CAD build for the part. Positions are in the model's coordinates, mm. Face numbers are marked on the shaded views. A direction names the side the tool comes from. Give positions to 0.01 mm unless a question says otherwise; leave off trailing zeros. Write each loop counter-clockwise with the first axis right and the second up, starting at its lowest first coordinate (ties: lowest second). Pieces come first, ordered by that corner, then holes. Notation, with made-up numbers: (37, 72) - (89, 72) arc R17 cw to (89, 102) - close; hole circle Ø5 at (71, 46). An arc over 180 degrees is marked (long way). Put each result on its own line as item: value. Start each with the question number.
1. Cut at D-D on x = 34. List the corners of the cut face in (y, z).
2. Wall check: line 1 (Y direction, x = 64, z = 27); line 2 (X direction, y = -10.5, z = 49); line 3 (X direction, y = -10.5, z = 110.5). Give the ranges that are in metal, low to high.
3. Drop flat-ended pins along their axis: pin 1 (16 mm diameter, centred on x = 16, y = 22, fed in from +Z); pin 2 (8 mm diameter, centred on x = -30, y = -41, fed in from +Z). Give the stop position or say it passes through.
4. Cut at C-C on z = 186. List the corners of the cut face in (x, y), and give its area (3 significant figures).
5. Tool access for the marked faces 1 and 2: list every direction of +Z, -Z, +X, -X, +Y, -Y with a clear straight run to the whole face (end or side of a thin tool).
6. Cut at B-B on z = 24. List the corners of the cut face in (x, y), and give its area (3 significant figures).
7. Cut at A-A on x = 0. List the corners of the cut face in (y, z) (3 decimals), and give its area (3 significant figures).
8. Mould opens along Y. For the marked faces 3, 4 and 5 say: +Y half, -Y half, draft (parallel to the pull), parting line (faces both ways), or undercut.
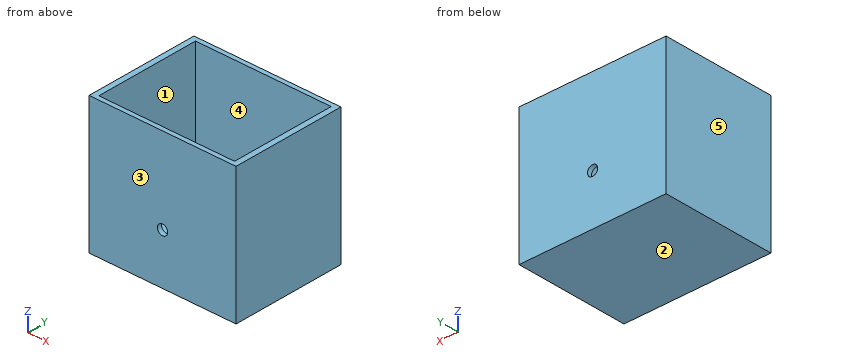
from build123d import *

# Parameters (mm, degrees)
SKETCH_W        = 216.32
SKETCH_H        = 167.18
PAD_DEPTH       = 200
SKETCH001_W     = 199.68
SKETCH001_H     = 154.08
POCKET_DEPTH    = 140
SKETCH002_W     = 166.5
SKETCH002_H     = 89
POCKET001_DEPTH = 30
SKETCH003_W     = 166.5
SKETCH003_H     = 20
POCKET002_DEPTH = 21
SKETCH004_R     = 7.5
HOLE_DEPTH      = 200


with BuildPart() as part:
    # Sketch → Pad (new body)
    with BuildSketch(Plane.XY):
        Rectangle(SKETCH_W, SKETCH_H)
    extrude(amount=PAD_DEPTH)

    # Sketch001 (on Face6 of Pad) → Pocket (cut)
    with BuildSketch(Plane.XY.offset(200)):
        Rectangle(SKETCH001_W, SKETCH001_H)
    extrude(amount=-POCKET_DEPTH, mode=Mode.SUBTRACT)

    # Sketch002 (on Face11 of Pocket) → Pocket001 (cut)
    with BuildSketch(Plane.XY.offset(60)):
        Rectangle(SKETCH002_W, SKETCH002_H)
    extrude(amount=-POCKET001_DEPTH, mode=Mode.SUBTRACT)

    # Sketch003 (on Face16 of Pocket001) → Pocket002 (cut)
    with BuildSketch(Plane.XY.offset(30)):
        with Locations((0, 24.5)):
            Rectangle(SKETCH003_W, SKETCH003_H)
        with Locations((0, -24.5)):
            Rectangle(SKETCH003_W, SKETCH003_H)
    extrude(amount=-POCKET002_DEPTH, mode=Mode.SUBTRACT)

    # Sketch004 (on Face6 of Pocket002) → Hole (cut)
    with BuildSketch(Plane.XZ.offset(83.59)):
        with Locations((0, 74.375)):
            Circle(SKETCH004_R)
    extrude(amount=-HOLE_DEPTH, mode=Mode.SUBTRACT)


solid = part.part
Report:
1. outline: (-83.59, 0) - (83.59, 0) - (83.59, 200) - (77.04, 200) - (77.04, 60) - (44.5, 60) - (44.5, 30) - (34.5, 30) - (34.5, 9) - (14.5, 9) - (14.5, 30) - (-14.5, 30) - (-14.5, 9) - (-34.5, 9) - (-34.5, 30) - (-44.5, 30) - (-44.5, 60) - (-77.04, 60) - (-77.04, 200) - (-83.59, 200) - close
2. line 1: y = -83.59 to -34.5, -14.5 to 14.5, 34.5 to 83.59
2. line 2: x = -108.16 to -83.25, 83.25 to 108.16
2. line 3: x = -108.16 to -99.84, 99.84 to 108.16
3. pin 1: stops at z = 30
3. pin 2: stops at z = 60
4. outline: (-108.16, -83.59) - (108.16, -83.59) - (108.16, 83.59) - (-108.16, 83.59) - close; hole (-99.84, -77.04) - (99.84, -77.04) - (99.84, 77.04) - (-99.84, 77.04) - close
4. area: 5,400 mm²
5. face 1: +Z
5. face 2: -Z, +X, -X, +Y, -Y
6. outline: (-108.16, -83.59) - (108.16, -83.59) - (108.16, 83.59) - (-108.16, 83.59) - close; hole (-83.25, -34.5) - (83.25, -34.5) - (83.25, -14.5) - (-83.25, -14.5) - close; hole (-83.25, 14.5) - (83.25, 14.5) - (83.25, 34.5) - (-83.25, 34.5) - close
6. area: 29,500 mm²
7. outline: (-83.59, 0) - (83.59, 0) - (83.59, 66.875) - (77.04, 66.875) - (77.04, 60) - (44.5, 60) - (44.5, 30) - (34.5, 30) - (34.5, 9) - (14.5, 9) - (14.5, 30) - (-14.5, 30) - (-14.5, 9) - (-34.5, 9) - (-34.5, 30) - (-44.5, 30) - (-44.5, 60) - (-77.04, 60) - (-77.04, 66.875) - (-83.59, 66.875) - close; (-83.59, 81.875) - (-77.04, 81.875) - (-77.04, 200) - (-83.59, 200) - close; (77.04, 81.875) - (83.59, 81.875) - (83.59, 200) - (77.04, 200) - close
7. area: 8,160 mm²
8. face 3: -Y half
8. face 4: undercut
8. face 5: draft
